Design review of the part built by this model. Coordinates are the model's own, in mm. Give positions to 0.01 mm unless a question says otherwise; leave off trailing zeros. Order: outer loops, then holes, each group sorted by start corner. A loop starts at its lowest first (then second) coordinate and runs counter-clockwise, first axis right, second up. Notation, with made-up numbers: M 30.5,-4 L 59.5,-4 A22 ccw 59.5,2 Z; hole C 84,63 d9. An arc over 180 degrees is marked long. Answer as a JSON object with one key per item and string values.
from build123d import *

# Parameters (mm, degrees)
CYLINDER006_R     = 2.75
CYLINDER006_DEPTH = 2


with BuildPart() as sphere005:
    # Sphere005 → Sphere005 (revolve)
    with BuildSketch(Plane(origin=(-6.25, 0, 15.25), x_dir=(1, 0, 0), z_dir=(0, -1, 0))):
        with BuildLine():
            ThreePointArc((0, -2.25), (2.25, 0), (0, 2.25))
            Line((0, 2.25), (0, -2.25))
        make_face()
    revolve(axis=Axis((-6.25, 0, 15.25), (0, 0, 1)))


with BuildPart() as cut003:
    # Cylinder006 → Cylinder006 (new body)
    with BuildSketch(Plane(origin=(-6.25, 0, 13), x_dir=(1, 0, 0), z_dir=(0, 0, 1))):
        Circle(CYLINDER006_R)
    extrude(amount=CYLINDER006_DEPTH)

    # Cut003: cut Sphere005
    add(sphere005.part, mode=Mode.SUBTRACT)


solid = cut003.part
(1) To check wall thickness, follow L1, parallel to Y at x = -7.15, z = 14.6; L2, parallel to X at y = 1.15, z = 14.75; L3, parallel to X at y = -1.8, z = 14.5. State the ranges of each line that lie inside material, in increasing order. Write a range as from..to.
Checked values:
{"L1": "y = -2.6..-1.96, 1.96..2.6", "L2": "x = -8.75..-8.12, -4.38..-3.75", "L3": "x = -8.33..-7.37, -5.13..-4.17"}
(2) We need section A-A (z = 13.95). Write out the cut boundary in (x, y).
Checked values:
{"outline": "C -6.25,0 d5.5; hole C -6.25,0 d3.67"}
(3) We need section D-D (z = 14.35). Write out the cut boundary in (x, y).
Checked values:
{"outline": "C -6.25,0 d5.5; hole C -6.25,0 d4.12"}
(4) We need section B-B (x = -7.65). Write out the cut boundary in (y, z).
Checked values:
{"outline": "M -2.37,13 L 2.37,13 L 2.37,15 L 1.74,15 A1.76 cw -1.74,15 L -2.37,15 Z"}
(5) Insertion check: pin 1 (1 mm diameter, centred on x = -4, z = 14.5, fed in from +Y); pin 2 (2 mm diameter, centred on x = -6.5, y = 0, fed in from +Z). Each pin has a flat end and moves straight along its axis. Give the tip position at first contact, or say it passes through.
Checked values:
{"pin 1": "stops at y = 2.12", "pin 2": "stops at z = 13.38"}
